Geometry check sheet. Reference: the model listing, model coordinates, mm. Round coordinates to 2 decimals unless told otherwise and drop trailing zeros. Order: outer loops, then holes, each group sorted by start corner. A loop starts at its lowest first (then second) coordinate and runs counter-clockwise, first axis right, second up.
Autodesk Inventor part; units mm, degrees
ref_plane "YZ Plane" through (0, 0, 0) normal (1, 0, 0) x (0, 1, 0)
ref_plane "XZ Plane" through (0, 0, 0) normal (0, 1, 0) x (-1, 0, 0)
ref_plane "XY Plane" through (0, 0, 0) normal (0, 0, 1) x (1, 0, 0)
sketch "Sketch1" plane through (0, 0, 0) normal (0, 0, 1) x (1, 0, 0)
  line L0 (0, 0) -> (30, 0)
  line L1 (30, 0) -> (30, 35)
  line L2 (30, 35) -> (0, 35)
  line L3 (0, 35) -> (0, 0)
  circle A0 centre (15, 17) radius 13
  dimension "d0" = 30
  dimension "d1" = 35
  dimension "d2" = 26
  dimension "d3" = 15
  dimension "d4" = 18
extrude "Extrusion1" add sketch "Sketch1" along normal blind 10
sketch "Sketch4" plane through (30, 0, 0) normal (1, 0, 0) x (0, 0, -1)
  line L0 (0, 0) -> (-10, 0)
  line L1 (0, 0) -> (0, 35)
  line L2 (-10, 0) -> (0, 0)
  line L3 (0, 0) -> (0, 18)
  line L4 (0, 18) -> (-10, 18)
  line L5 (-10, 18) -> (-10, 0)
  dimension "d25" = 18
extrude "Extrusion2" cut sketch "Sketch4" against normal through all
sketch "Sketch5" plane through (30, 35, 10) normal (1, 0, 0) x (0, 0, -1)
  line L0 (10, 0) -> (10, -17)
  line L1 (0, 0) -> (0, -17)
  line L2 (10, -17) -> (0, -17)
  line L3 (0, -17) -> (0, 0)
  line L4 (0, 0) -> (10, 0)
  line L5 (10, 0) -> (10, -17)
  point P0 (10, -35)
extrude "Extrusion3" add sketch "Sketch5" along normal blind 10
sketch "Sketch6" plane through (0, 35, 0) normal (-1, 0, 0) x (0, 0, 1)
  line L0 (0, -17) -> (0, 0)
  line L1 (10, -17) -> (0, -17)
  line L2 (0, -17) -> (0, 0)
  line L3 (0, 0) -> (10, 0)
  line L4 (10, 0) -> (10, -17)
  point P0 (0, -35)
extrude "Extrusion4" add sketch "Sketch6" along normal blind 10
sketch "Sketch7" plane through (40, 35, 10) normal (0, 1, 0) x (1, 0, 0)
  circle A0 centre (-45, 5) radius 1.75
  circle A1 centre (-5, 5) radius 1.75
  line L0 (-50, 0) -> (-50, 10)
  line L1 (-50, 10) -> (0, 10)
  line L2 (0, 10) -> (0, 0)
  point P0 (-40, 10)
  dimension "d32" = 3.5
  dimension "d33" = 3.5
  dimension "d34" = 5
  dimension "d35" = 5
  dimension "d36" = 5
  dimension "d37" = 5
extrude "Extrusion5" cut sketch "Sketch7" against normal through all
properties part number "motortarto" material "ABS Plastic"
(1) Sectioned sample at D-D, the plane y = 32.5. Record the cut outline in (x, z).
Returned:
outline: (-10, 0) - (40, 0) - (40, 10) - (-10, 10) - close; hole circle Ø3.5 at (-5, 5); hole circle Ø3.5 at (35, 5)
(2) Sectioned sample at B-B, the plane y = 22.25. Record the cut outline in (x, z).
Returned:
outline: (-10, 0) - (3.11, 0) - (3.11, 10) - (-10, 10) - close; (26.89, 0) - (40, 0) - (40, 10) - (26.89, 10) - close; hole circle Ø3.5 at (-5, 5); hole circle Ø3.5 at (35, 5)
(3) Sectioned sample at A-A, the plane x = -5. Record the cut outline in (y, z), and give its area (4 significant figures).
Returned:
outline: (18, 0) - (35, 0) - (35, 3.25) - (18, 3.25) - close; (18, 6.75) - (35, 6.75) - (35, 10) - (18, 10) - close
area: 110.5 mm2
(4) Material ranges on line 1 (X direction, y = 31.5, z = 5); line 2 (Z direction, x = 35, y = 28.75); line 3 (X direction, y = 22.5, z = 3.75), recorded low to high.
Returned:
line 1: x = -10 to -6.75, -3.25 to 33.25, 36.75 to 40
line 2: z = 0 to 3.25, 6.75 to 10
line 3: x = -10 to -6.22, -3.78 to 3.22, 26.78 to 33.78, 36.22 to 40
(5) Depth check by flat-ended pin: P1, Ø2, axis at x = 28, y = 33, coming from the -Z side. Enter the tip coordinate at first touch or a pass-through.
Returned:
P1: stops at z = 0
(6) Draft check along Z on faces 1 (the flat face through (15.4, 30.4, 10)), 2 (the cylindrical face through (33.61, 26.62, 6.06)), 3 (the flat face through (-3, 18, 5)). Enter one of: released by +Z, released by -Z, zero draft, split by the parting line, or undercut.
Returned:
face 1: released by +Z
face 2: undercut
face 3: zero draft
(7) Sectioned sample at C-C, the plane z = 5. Record the cut outline in (x, y).
Returned:
outline: (-10, 18) - (-6.75, 18) - (-6.75, 35) - (-10, 35) - close; (-3.25, 18) - (2.04, 18) arc R13 cw to (27.96, 18) - (33.25, 18) - (33.25, 35) - (-3.25, 35) - close; (36.75, 18) - (40, 18) - (40, 35) - (36.75, 35) - close
